```python
from build123d import *

# Parameters (mm, degrees)
SKETCH3_R           = 10
BOSS_EXTRUDE4_DEPTH = 35
FILLET3_R           = 10
CUT_EXTRUDE1_DEPTH  = 12
CUT_EXTRUDE2_DEPTH  = 22.5
FILLET4_R           = 25
FILLET5_R           = 10
CHAMFER2_SIZE       = 5
CHAMFER4_SIZE       = 5


with BuildPart() as part:
    # Sketch3 → Boss-Extrude4 (new body)
    with BuildSketch(Plane.XY):
        with BuildLine():
            Line((-25, 0), (-25, -11.491470389))
            Line((-25, -11.491470389), (-63.508529611, -50))
            Line((-63.508529611, -50), (-25.980762114, -115))
            ThreePointArc((-25.980762114, -115), (0, -130), (25.980762114, -115))
            Line((25.980762114, -115), (63.508529611, -50))
            Line((63.508529611, -50), (25, -11.491470389))
            Line((25, -11.491470389), (25, 0))
            ThreePointArc((25, 0), (0, 25), (-25, 0))
        make_face()
        Circle(SKETCH3_R, mode=Mode.SUBTRACT)
        with Locations((0, -100)):
            Circle(SKETCH3_R, mode=Mode.SUBTRACT)
    extrude(amount=BOSS_EXTRUDE4_DEPTH)

    # Fillet3
    fillet3_edges = [part.edges().sort_by_distance(p)[0] for p in [
        (-63.508529611, -50, 17.5),
        (63.508529611, -50, 17.5),
    ]]
    fillet(fillet3_edges, radius=FILLET3_R)

    # Sketch5 → Cut-Extrude1 (cut)
    with BuildSketch(Plane(origin=(0, 0, 0), x_dir=(-1, 0, 0), z_dir=(0, 0, -1))):
        with BuildLine():
            Line((-53.508529611, -40), (53.508529611, -40))
            Line((53.508529611, -40), (25, -11.491470389))
            Line((25, -11.491470389), (25, 0))
            ThreePointArc((25, 0), (0, 25), (-25, 0))
            Line((-25, 0), (-25, -11.491470389))
            Line((-25, -11.491470389), (-53.508529611, -40))
        make_face()
    extrude(amount=-CUT_EXTRUDE1_DEPTH, mode=Mode.SUBTRACT)

    # Sketch6 → Cut-Extrude2 (cut)
    with BuildSketch(Plane.XY.offset(35)):
        with BuildLine():
            Line((-51.508529611, -38), (51.508529611, -38))
            Line((51.508529611, -38), (58.082708445, -44.574178834))
            ThreePointArc((58.082708445, -44.574178834), (60.926089247, -50.339984724), (59.671894671, -56.645246646))
            Line((59.671894671, -56.645246646), (25.980762114, -115))
            ThreePointArc((25.980762114, -115), (0, -130), (-25.980762114, -115))
            Line((-25.980762114, -115), (-59.671894671, -56.645246646))
            ThreePointArc((-59.671894671, -56.645246646), (-60.926089247, -50.339984724), (-58.082708445, -44.574178834))
            Line((-58.082708445, -44.574178834), (-51.508529611, -38))
        make_face()
    extrude(amount=-CUT_EXTRUDE2_DEPTH, mode=Mode.SUBTRACT)

    # Fillet4
    # the kernel refuses this fillet: 25 mm, written as the material it adds along each edge
    with BuildSketch(Plane(origin=(106.893920871, -40, 12), x_dir=(0, 1, 0), z_dir=(-1, 0, 0))) as fillet4_piece_1_section:
        with BuildLine():
            CenterArc((21.354156504, 25), FILLET4_R, 211.332251498, 58.667748502)
            Line((0, 12), (-0.42708313, 11.74))
            ThreePointArc((-0.42708313, 11.74), (-0.5, 6), (-0.5, 0))
            Line((-0.5, 0), (0, -0.5))
            Line((0, -0.5), (21.354156504, -0.5))
            Line((21.354156504, -0.5), (21.354156504, 0))
        make_face()
    fillet4_piece_1 = extrude(amount=213.787841742, mode=Mode.PRIVATE)
    fillet4_piece_1 = split(fillet4_piece_1, bisect_by=Plane(origin=(-24.314247143, -10.805717532, 8.724953467), z_dir=(0.7071067811865464, -0.7071067811865487, 0)), keep=Keep.TOP, mode=Mode.PRIVATE)
    fillet4_piece_1 = split(fillet4_piece_1, bisect_by=Plane(origin=(24.314247143, -10.805717532, 8.724953467), z_dir=(-0.7071067811865461, -0.7071067811865489, 0)), keep=Keep.TOP, mode=Mode.PRIVATE)
    add(fillet4_piece_1)

    # Fillet5
    fillet5_edges = [part.edges().sort_by_distance(p)[0] for p in [
        (0, -38, 12.5),
    ]]
    fillet(fillet5_edges, radius=FILLET5_R)

    # Chamfer2
    chamfer2_edges = [part.edges().sort_by_distance(p)[0] for p in [
        (-10, 0, 12),
    ]]
    chamfer(chamfer2_edges, length=CHAMFER2_SIZE)

    # Mirror2: part across plane


with BuildPart() as part_1:
    add(part.part)
    add(part.part.mirror(Plane(origin=(0, -100, 35), x_dir=(1, 0, 0), z_dir=(0, 0, 1))))

    # Chamfer4
    chamfer4_edges = [part_1.edges().sort_by_distance(p)[0] for p in [
        (-10, -100, 70),
        (-10, -100, 0),
    ]]
    chamfer(chamfer4_edges, length=CHAMFER4_SIZE)


solid = part_1.part
```
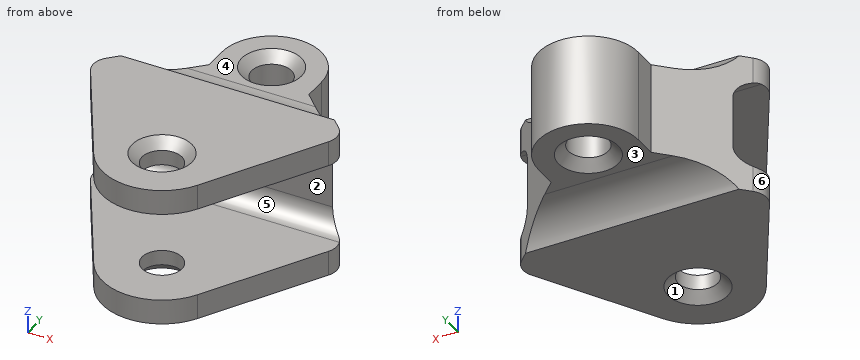
Part model, mm, in its own coordinate system. Face numbers are marked on the shaded views. A direction names the side the tool comes from. Round coordinates to 2 decimals unless told otherwise and drop trailing zeros. Order: outer loops, then holes, each group sorted by start corner. A loop starts at its lowest first (then second) coordinate and runs counter-clockwise, first axis right, second up. Notation, with made-up numbers: M -33,79 L 22,79 A32 ccw 22,111 Z; hole C -24,35 d1. An arc over 180 degrees is marked long. Put each result on its own line as item: value. Start each with the question number.
1. Drill centre lines: probe 1 along Z at (x, y) = (-15.5, -123); probe 2 along Y at (x, z) = (0, 25); probe 3 along Z at (x, y) = (31.5, -19). Where is each one in solid material? Low to high. Write a range as [from, to].
2. Slice it at B-B on z = 40. List the corners of the cut face in (x, y).
3. Drop flat-ended pins along their axis: pin 1 (1.5 mm diameter, centred on x = -16, y = -13, fed in from -Z); pin 2 (3 mm diameter, centred on y = -8.5, z = 29.5, fed in from -X); pin 3 (5.5 mm diameter, centred on y = -7, z = 40, fed in from +X). Give the stop position or say it passes through.
4. Slice it at D-D on y = -22. List the corners of the cut face in (x, z).
5. Tool access for the marked faces 1, 2 and 3: list every direction of +Z, -Z, +X, -X, +Y, -Y with a clear straight run to the whole face (end or side of a thin tool).
6. Slice it at A-A on x = 0. State how many separate pieces and enclosed holes the cut face has, then the cut area to 3 significant figures.
7. Slice it at C-C on y = -100. List the corners of the cut face in (x, z), then the cut area to 3 significant figures.
8. Two-plate mould, pull along Z, no slides. Class the marked faces 4, 5 and 6: +Z half, -Z half, draft (parallel to the pull), parting line (faces both ways), or undercut.
Findings:
1. probe 1: [0, 12.5], [57.5, 70]
1. probe 2: [-38, -10], [10, 25]
1. probe 3: [12, 58]
2. outline: M -51.51,-38 L 51.51,-38 L 25,-11.49 L 25,0 A25 ccw -25,0 L -25,-11.49 Z; hole C 0,0 d20
3. pin 1: z = 12
3. pin 2: x = -25
3. pin 3: x = 25
4. outline: M -35.51,11.77 L 35.51,11.77 L 35.51,58.23 L -35.51,58.23 Z
5. face 1: -Z
5. face 2: +X, -X, -Y
5. face 3: -Z, +X, -X, +Y
6. separate pieces: 4
6. enclosed holes: 0
6. area: 3,820 mm2
7. outline: M -34.64,0 L -15,0 L -10,5 L -10,12.5 L -34.64,12.5 Z; M -34.64,57.5 L -10,57.5 L -10,65 L -15,70 L -34.64,70 Z; M 10,5 L 15,0 L 34.64,0 L 34.64,12.5 L 10,12.5 Z; M 10,57.5 L 34.64,57.5 L 34.64,70 L 15,70 L 10,65 Z
7. area: 1,180 mm2
8. face 4: +Z half
8. face 5: undercut
8. face 6: draft
